For this review, take the finished solid that the model builds, in its own axes (mm). A direction names the side the tool comes from. Give positions to 0.01 mm unless a question says otherwise; leave off trailing zeros. Loops run counter-clockwise (first coordinate to the right, second up) from the corner with the lowest first, then second, coordinate; pieces in that order, holes last.
Autodesk Inventor part; units mm, degrees
ref_plane "dia1_XY" through (-6.35, 5.5499, 0) normal (1, 0, 0) x (0, 0, -1)
ref_plane "dia1_YZ" through (-6.35, 5.5499, 0) normal (0, 0, -1) x (0, 1, 0)
ref_plane "dia1_ZX" through (-6.35, 5.5499, 0) normal (0, 1, 0) x (1, 0, 0)
sketch "Sketch_1" plane through (0, 0, 0) normal (0, 0, 1) x (1, 0, 0)
  line L0 (222.377, 0) -> (-6.35, 0)
  line L1 (-6.35, 0) -> (-6.35, 5.5499)
  line L2 (-6.35, 5.5499) -> (200.025, 5.5499)
  line L3 (200.025, 5.5499) -> (200.025, 19.1453)
  line L4 (200.025, 19.1453) -> (222.377, 19.1453)
  line L5 (222.377, 19.1453) -> (222.377, 0)
  line L6 (222.377, 0) -> (-6.35, 0)
revolve "Revolution1" add sketch "Sketch_1" angle 360 about axis through (222.377, 0, 0) along (1, 0, 0)
sketch "Sketch_3" plane through (0, 0, 0) normal (0, 0, 1) x (1, 0, 0)
  line L0 (-6.35, 0) -> (-25.4, 0)
  line L1 (-25.4, 0) -> (-25.4, 4.8006)
  line L2 (-25.4, 4.8006) -> (-24.6443, 5.5563)
  line L3 (-24.6443, 5.5563) -> (-6.35, 5.5563)
  line L4 (-6.35, 5.5563) -> (-6.35, 0)
  line L5 (-6.35, 0) -> (-25.4, 0)
revolve "Revolution2" add sketch "Sketch_3" angle 360 about axis through (-6.35, 0, 0) along (1, 0, 0)
thread "Thread1"
sketch "Sketch_10" plane through (-6.35, 0, 0) normal (1, 0, 0) x (0, 0, -1)
  line L0 (-11.0998, -11.0998) -> (11.0998, -11.0998)
  line L1 (11.0998, -11.0998) -> (11.0998, 11.0998)
  line L2 (11.0998, 11.0998) -> (-11.0998, 11.0998)
  line L3 (-11.0998, 11.0998) -> (-11.0998, -11.0998)
  line L4 (-4.826, -5.5499) -> (4.826, -5.5499)
  line L5 (4.826, -5.5499) -> (4.826, 5.5499)
  line L6 (4.826, 5.5499) -> (-4.826, 5.5499)
  line L7 (-4.826, 5.5499) -> (-4.826, -5.5499)
extrude "Extrusion1" cut sketch "Sketch_10" along normal blind 6.35
ref_plane "dia1_XY" through (-6.35, 5.5499, 0) normal (1, 0, 0) x (0, 0, -1)
ref_plane "dia1_YZ" through (-6.35, 5.5499, 0) normal (0, 0, -1) x (0, 1, 0)
ref_plane "dia1_ZX" through (-6.35, 5.5499, 0) normal (0, 1, 0) x (1, 0, 0)
ref_plane "dia12_XY" through (0, 0, 19.7675) normal (1, 0, 0) x (0, 0, -1)
ref_plane "dia12_YZ" through (0, 0, 19.7675) normal (0, 0, -1) x (0, 1, 0)
ref_plane "dia12_ZX" through (0, 0, 19.7675) normal (0, 1, 0) x (1, 0, 0)
ref_plane "dia2_XY" through (-6.35, -5.5499, 0) normal (1, 0, 0) x (0, 0, -1)
ref_plane "dia2_YZ" through (-6.35, -5.5499, 0) normal (0, 0, -1) x (0, 1, 0)
ref_plane "dia2_ZX" through (-6.35, -5.5499, 0) normal (0, 1, 0) x (1, 0, 0)
ref_plane "dia22_XY" through (0, 0, -19.7675) normal (1, 0, 0) x (0, 0, -1)
ref_plane "dia22_YZ" through (0, 0, -19.7675) normal (0, 0, -1) x (0, 1, 0)
ref_plane "dia22_ZX" through (0, 0, -19.7675) normal (0, 1, 0) x (1, 0, 0)
ref_plane "rl1_XY" through (-25.4, 0, 0) normal (1, 0, 0) x (0, 0, -1)
ref_plane "rl1_YZ" through (-25.4, 0, 0) normal (0, 0, -1) x (0, 1, 0)
ref_plane "rl1_ZX" through (-25.4, 0, 0) normal (0, 1, 0) x (1, 0, 0)
ref_plane "rl2_XY" through (-6.35, 0, 0) normal (1, 0, 0) x (0, 0, -1)
ref_plane "rl2_YZ" through (-6.35, 0, 0) normal (0, 0, -1) x (0, 1, 0)
ref_plane "rl2_ZX" through (-6.35, 0, 0) normal (0, 1, 0) x (1, 0, 0)
ref_plane "rod_cp_XY" through (0, 0, 0) normal (1, 0, 0) x (0, 0, -1)
ref_plane "rod_cp_YZ" through (0, 0, 0) normal (0, 0, -1) x (0, 1, 0)
ref_plane "rod_cp_ZX" through (0, 0, 0) normal (0, 1, 0) x (1, 0, 0)
ref_plane "thd1_XY" through (-25.4, 5.5563, 0) normal (1, 0, 0) x (0, 0, -1)
ref_plane "thd1_YZ" through (-25.4, 5.5563, 0) normal (0, 0, -1) x (0, 1, 0)
ref_plane "thd1_ZX" through (-25.4, 5.5563, 0) normal (0, 1, 0) x (1, 0, 0)
ref_plane "thd2_XY" through (-25.4, -5.5563, 0) normal (1, 0, 0) x (0, 0, -1)
ref_plane "thd2_YZ" through (-25.4, -5.5563, 0) normal (0, 0, -1) x (0, 1, 0)
ref_plane "thd2_ZX" through (-25.4, -5.5563, 0) normal (0, 1, 0) x (1, 0, 0)
ref_plane "to_rod_clevis_XY" through (-30.988, 0, 0) normal (1, 0, 0) x (0, 0, -1)
ref_plane "to_rod_clevis_YZ" through (-30.988, 0, 0) normal (0, 0, -1) x (0, 1, 0)
ref_plane "to_rod_clevis_ZX" through (-30.988, 0, 0) normal (0, 1, 0) x (1, 0, 0)
ref_plane "wf1_XY" through (-6.35, 0, 0) normal (1, 0, 0) x (0, 0, -1)
ref_plane "wf1_YZ" through (-6.35, 0, 0) normal (0, 0, -1) x (0, 1, 0)
ref_plane "wf1_ZX" through (-6.35, 0, 0) normal (0, 1, 0) x (1, 0, 0)
ref_plane "wf2_XY" through (0, 0, 0) normal (1, 0, 0) x (0, 0, -1)
ref_plane "wf2_YZ" through (0, 0, 0) normal (0, 0, -1) x (0, 1, 0)
ref_plane "wf2_ZX" through (0, 0, 0) normal (0, 1, 0) x (1, 0, 0)
ref_plane "wfw1_XY" through (-6.35, 0, -4.826) normal (0, 1, 0) x (1, 0, 0)
ref_plane "wfw1_YZ" through (-6.35, 0, -4.826) normal (1, 0, 0) x (0, 0, -1)
ref_plane "wfw1_ZX" through (-6.35, 0, -4.826) normal (0, 0, -1) x (0, 1, 0)
ref_plane "wfw2_XY" through (-6.35, 0, 4.826) normal (0, 1, 0) x (1, 0, 0)
ref_plane "wfw2_YZ" through (-6.35, 0, 4.826) normal (1, 0, 0) x (0, 0, -1)
ref_plane "wfw2_ZX" through (-6.35, 0, 4.826) normal (0, 0, -1) x (0, 1, 0)
properties part number "C-176-DP0000_rod"
Q1. Consider section B-B on y = 0. Give the boundary of the cut face in (x, z) (3 decimals).
Answers:
outline: (-25.4, -4.801) - (-24.644, -5.556) - (-6.35, -5.556) - (-6.35, -4.826) - (0, -4.826) - (0, -5.55) - (200.025, -5.55) - (200.025, -19.145) - (222.377, -19.145) - (222.377, 19.145) - (200.025, 19.145) - (200.025, 5.55) - (0, 5.55) - (0, 4.826) - (-6.35, 4.826) - (-6.35, 5.556) - (-24.644, 5.556) - (-25.4, 4.801) - close
Q2. Consider section D-D on z = -9.5. Give the boundary of the cut face in (x, y) (3 decimals).
Answers:
outline: (200.025, -16.622) - (222.377, -16.622) - (222.377, 16.622) - (200.025, 16.622) - close
Q3. Mouldability with a two-part tool opening along X and no side actions: class faces 4 (the cylindrical face through (98.282, 5.127, -2.126)), 5 (the flat face through (-3, 0, 4.826)), 6 (the flat face through (-25.4, 0, 0)) as +X half, -X half, draft (parallel to the pull), parting line (faces both ways), or undercut.
Answers:
face 4: draft
face 5: undercut
face 6: -X half
Q4. Consider section A-A on z = 0. Give the boundary of the cut face in (x, y) (3 decimals), plus the area to 3 significant figures.
Answers:
outline: (-25.4, -4.801) - (-24.644, -5.556) - (-6.35, -5.556) - (-6.35, -5.55) - (200.025, -5.55) - (200.025, -19.145) - (222.377, -19.145) - (222.377, 19.145) - (200.025, 19.145) - (200.025, 5.55) - (-6.35, 5.55) - (-6.35, 5.556) - (-24.644, 5.556) - (-25.4, 4.801) - close
area: 3,360 mm2
Q5. For pin 1 Ø1.5 at (x, z) = (6.5, -5) entering from -Y; pin 2 Ø1.6 at (x, y) = (-2, 1) entering from +Z; pin 3 Ø1.5 at (y, z) = (-1, 13) entering from -X (3 decimals); pin 4 Ø0.8 at (y, z) = (0, -5) entering from -X, all flat-tipped, find the tip position at first contact; note any pin that passes through.
Answers:
pin 1: stops at y = -3.57
pin 2: stops at z = 4.83
pin 3: stops at x = 200.025
pin 4: stops at x = -25.4
Q6. For probe 1 along Z at (x, y) = (61, 0); probe 2 along Z at (x, y) = (204, 1); probe 3 along X at (y, z) = (-6.5, -4.5) (3 decimals), list the stretches that pass through material, from the lowest coordinate up.
Answers:
probe 1: z = -5.55 to 5.55
probe 2: z = -19.12 to 19.12
probe 3: x = 200.025 to 222.377
Q7. Consider section C-C on x = 3. Give the boundary of the cut face in (y, z), plus the area to 3 significant figures.
Answers:
outline: circle Ø11.1 at (0, 0)
area: 96.8 mm2
Q8. Machinability: for faces 1 (the flat face through (222.377, 0, 0)), 2 (the flat face through (-3, 0, -4.826)), 3 (the flat face through (200.025, 4, 5)), which of the approach directions +Z, -Z, +X, -X, +Y, -Y give a long, thin tool a straight path to every point of the face, cutting with its end or side? Answer none if there is none.
Answers:
face 1: +Z, -Z, +X, +Y, -Y
face 2: -Z, +Y, -Y
face 3: -X
